Check sheet for the modelled part. Datum: model origin and axes. Units: mm. A direction names the side the tool comes from. Round coordinates to 2 decimals unless told otherwise and drop trailing zeros. Loops run counter-clockwise (first coordinate to the right, second up) from the corner with the lowest first, then second, coordinate; pieces in that order, holes last. Notation, with made-up numbers: (63.5, 37) -> (76.5, 37) arc R21 ccw to (76.5, 71) -> close; hole circle Ø8 at (79.25, 88.5). An arc over 180 degrees is marked (long way). One line per question, with ' | ' between items.
```python
from build123d import *

# Parameters (mm, degrees)
F1_DEPTH = 6


with BuildPart() as f1:
    # F0 (on Right) → F1 (new body)
    with BuildSketch(Plane.YZ):
        with BuildLine():
            Line((-160, 0), (-1.27, 0))
            ThreePointArc((-1.27, 0), (-0.371974, 0.371974), (0, 1.27))
            Line((0, 1.27), (0, 240))
            Line((0, 240), (0, 248.73))
            ThreePointArc((0, 248.73), (-0.371974, 249.628026), (-1.27, 250))
            Line((-1.27, 250), (-158.73, 250))
            ThreePointArc((-158.73, 250), (-159.628026, 249.628026), (-160, 248.73))
            Line((-160, 248.73), (-160, 120))
            Line((-160, 120), (-160, 105))
            ThreePointArc((-160, 105), (-120, 65), (-160, 25))
            Line((-160, 25), (-160, 0))
        make_face()
        with BuildLine():
            Line((0, 248.73), (0, 240))
            Line((0, 240), (10, 240))
            Line((10, 240), (10, 225))
            Line((10, 225), (20, 225))
            Line((20, 225), (20, 270))
            Line((20, 270), (-180, 270))
            Line((-180, 270), (-180, 105))
            Line((-180, 105), (-170, 105))
            Line((-170, 105), (-170, 120))
            Line((-170, 120), (-160, 120))
            Line((-160, 120), (-160, 248.73))
            ThreePointArc((-160, 248.73), (-159.628026, 249.628026), (-158.73, 250))
            Line((-158.73, 250), (-1.27, 250))
            ThreePointArc((-1.27, 250), (-0.371974, 249.628026), (0, 248.73))
        make_face()
    extrude(amount=F1_DEPTH)


solid = f1.part
```
(1) Go/stop test with flat-tipped pins: pin 1 (1.8 mm diameter, centred on x = 3, y = -166, fed in from -Z); pin 2 (2 mm diameter, centred on x = 4, z = 29, fed in from +Y); pin 3 (1.8 mm diameter, centred on x = 4.5, y = 13, fed in from -Z). Record where each tip stops, or that it passes through.
Answer:
pin 1: stops at z = 120 | pin 2: stops at y = 0 | pin 3: stops at z = 225
(2) Set-up check for faces 1 (the face through (3, 20, 247)), 2 (the face through (0, -81, 137)), 3 (the face through (3, 15, 225)), 4 (the face through (3, -170, 112)), 5 (the face through (3, -175, 105)): record each of +Z, -Z, +X, -X, +Y, -Y from which the full face is reachable in a straight line by a thin tool's end or side.
Answer:
face 1: +Z, -Z, +X, -X, +Y | face 2: +Z, -Z, -X, +Y, -Y | face 3: -Z, +X, -X, +Y | face 4: -Z, +X, -X | face 5: -Z, +X, -X, -Y
(3) Mould release check, pull along Y, two halves, no side actions. Record for faces 6 (the face through (3, 5, 240)), 7 (the face through (2.96, -120.01, 65.88)), 8 (the face through (3, -79, 270)): +Y half, -Y half, draft (parallel to the pull), parting line (faces both ways), or undercut.
Answer:
face 6: undercut | face 7: -Y half | face 8: draft
(4) Sectioned sample at D-D, the plane z = 20. Record the cut outline in (x, y).
Answer:
outline: (0, -160) -> (6, -160) -> (6, 0) -> (0, 0) -> close
(5) Scan lines: probe 1 along Y at (x, z) = (3.25, 107.5); probe 2 along Z at (x, y) = (0.55, 2); probe 3 along Y at (x, z) = (1.2, 234.5). Record each from-to range of solid material in increasing order.
Answer:
probe 1: y = -180 to -170, -160 to 0 | probe 2: z = 240 to 270 | probe 3: y = -180 to 0, 10 to 20
(6) Sectioned sample at B-B, the plane y = -139.5. Record the cut outline in (x, z).
Answer:
outline: (0, 0) -> (6, 0) -> (6, 30.65) -> (0, 30.65) -> close; (0, 99.35) -> (6, 99.35) -> (6, 270) -> (0, 270) -> close
(7) Sectioned sample at C-C, the plane z = 65. Record the cut outline in (x, y).
Answer:
outline: (0, -120) -> (6, -120) -> (6, 0) -> (0, 0) -> close
(8) Sectioned sample at A-A, the plane x = 3. Record the cut outline in (y, z), and give its area (3 significant figures).
Answer:
outline: (-180, 105) -> (-170, 105) -> (-170, 120) -> (-160, 120) -> (-160, 105) arc R40 cw to (-160, 25) -> (-160, 0) -> (-1.27, 0) arc R1.27 ccw to (0, 1.27) -> (0, 240) -> (10, 240) -> (10, 225) -> (20, 225) -> (20, 270) -> (-180, 270) -> close | area: 44,600 mm2
